from build123d import *

# Parameters (mm, degrees)
F1_DEPTH = 25.4


with BuildPart() as f1:
    # F0 (on Front) → F1 (new body)
    with BuildSketch(Plane.XZ):
        with BuildLine():
            Line((-1.5875, 27.281528), (-2.760676, 25.249528))
            ThreePointArc((-2.760676, 25.249528), (-4.410664, 25.014117), (-6.041661, 24.671002))
            ThreePointArc((-6.041661, 24.671002), (-8.687312, 23.868193), (-11.230034, 22.782589))
            ThreePointArc((-11.230034, 22.782589), (-12.7, 21.997045), (-14.115283, 21.116789))
            ThreePointArc((-14.115283, 21.116789), (-16.326805, 19.457529), (-18.344884, 17.567733))
            ThreePointArc((-18.344884, 17.567733), (-19.457529, 16.326805), (-20.486395, 15.015579))
            ThreePointArc((-20.486395, 15.015579), (-21.997045, 12.7), (-23.247071, 10.233949))
            ThreePointArc((-23.247071, 10.233949), (-23.868193, 8.687312), (-24.386545, 7.103269))
            ThreePointArc((-24.386545, 7.103269), (-25.014117, 4.410664), (-25.345317, 1.6658))
            ThreePointArc((-25.345317, 1.6658), (-25.4, 0), (-25.345317, -1.6658))
            ThreePointArc((-25.345317, -1.6658), (-25.014117, -4.410664), (-24.386545, -7.103269))
            ThreePointArc((-24.386545, -7.103269), (-23.868193, -8.687312), (-23.247071, -10.233949))
            ThreePointArc((-23.247071, -10.233949), (-21.997045, -12.7), (-20.486395, -15.015579))
            ThreePointArc((-20.486395, -15.015579), (-19.457529, -16.326805), (-18.344884, -17.567733))
            ThreePointArc((-18.344884, -17.567733), (-16.326805, -19.457529), (-14.115283, -21.116789))
            ThreePointArc((-14.115283, -21.116789), (-12.7, -21.997045), (-11.230034, -22.782589))
            ThreePointArc((-11.230034, -22.782589), (-8.687312, -23.868193), (-6.041661, -24.671002))
            ThreePointArc((-6.041661, -24.671002), (-4.410664, -25.014117), (-2.760676, -25.249528))
            ThreePointArc((-2.760676, -25.249528), (0, -25.4), (2.760676, -25.249528))
            ThreePointArc((2.760676, -25.249528), (4.410664, -25.014117), (6.041661, -24.671002))
            ThreePointArc((6.041661, -24.671002), (8.687312, -23.868193), (11.230034, -22.782589))
            ThreePointArc((11.230034, -22.782589), (12.7, -21.997045), (14.115283, -21.116789))
            ThreePointArc((14.115283, -21.116789), (16.326805, -19.457529), (18.344884, -17.567733))
            ThreePointArc((18.344884, -17.567733), (19.457529, -16.326805), (20.486395, -15.015579))
            ThreePointArc((20.486395, -15.015579), (21.997045, -12.7), (23.247071, -10.233949))
            ThreePointArc((23.247071, -10.233949), (23.868193, -8.687312), (24.386545, -7.103269))
            ThreePointArc((24.386545, -7.103269), (25.014117, -4.410664), (25.345317, -1.6658))
            ThreePointArc((25.345317, -1.6658), (25.4, 0), (25.345317, 1.6658))
            ThreePointArc((25.345317, 1.6658), (25.014117, 4.410664), (24.386545, 7.103269))
            ThreePointArc((24.386545, 7.103269), (23.868193, 8.687312), (23.247071, 10.233949))
            ThreePointArc((23.247071, 10.233949), (21.997045, 12.7), (20.486395, 15.015579))
            ThreePointArc((20.486395, 15.015579), (19.457529, 16.326805), (18.344884, 17.567733))
            ThreePointArc((18.344884, 17.567733), (16.326805, 19.457529), (14.115283, 21.116789))
            ThreePointArc((14.115283, 21.116789), (12.7, 21.997045), (11.230034, 22.782589))
            ThreePointArc((11.230034, 22.782589), (8.687312, 23.868193), (6.041661, 24.671002))
            ThreePointArc((6.041661, 24.671002), (4.410664, 25.014117), (2.760676, 25.249528))
            Line((2.760676, 25.249528), (1.5875, 27.281528))
            Line((1.5875, 27.281528), (-1.5875, 27.281528))
        make_face()
        with BuildLine():
            ThreePointArc((-11.230034, 22.782589), (-8.687312, 23.868193), (-6.041661, 24.671002))
            Line((-6.041661, 24.671002), (-7.83907, 26.179208))
            Line((-7.83907, 26.179208), (-10.822594, 25.093294))
            Line((-10.822594, 25.093294), (-11.230034, 22.782589))
        make_face()
        with BuildLine():
            ThreePointArc((-18.344884, 17.567733), (-16.326805, 19.457529), (-14.115283, 21.116789))
            Line((-14.115283, 21.116789), (-16.320133, 21.919288))
            Line((-16.320133, 21.919288), (-18.752324, 19.878438))
            Line((-18.752324, 19.878438), (-18.344884, 17.567733))
        make_face()
        with BuildLine():
            Line((7.83907, 26.179208), (6.041661, 24.671002))
            ThreePointArc((6.041661, 24.671002), (8.687312, 23.868193), (11.230034, 22.782589))
            Line((11.230034, 22.782589), (10.822594, 25.093294))
            Line((10.822594, 25.093294), (7.83907, 26.179208))
        make_face()
        with BuildLine():
            ThreePointArc((-23.247071, 10.233949), (-21.997045, 12.7), (-20.486395, 15.015579))
            Line((-20.486395, 15.015579), (-22.832746, 15.015579))
            Line((-22.832746, 15.015579), (-24.420246, 12.265949))
            Line((-24.420246, 12.265949), (-23.247071, 10.233949))
        make_face()
        with BuildLine():
            Line((16.320133, 21.919288), (14.115283, 21.116789))
            ThreePointArc((14.115283, 21.116789), (16.326805, 19.457529), (18.344884, 17.567733))
            Line((18.344884, 17.567733), (18.752324, 19.878438))
            Line((18.752324, 19.878438), (16.320133, 21.919288))
        make_face()
        with BuildLine():
            ThreePointArc((-25.345317, 1.6658), (-25.014117, 4.410664), (-24.386545, 7.103269))
            Line((-24.386545, 7.103269), (-26.591394, 6.30077))
            Line((-26.591394, 6.30077), (-27.142727, 3.174005))
            Line((-27.142727, 3.174005), (-25.345317, 1.6658))
        make_face()
        with BuildLine():
            Line((22.832746, 15.015579), (20.486395, 15.015579))
            ThreePointArc((20.486395, 15.015579), (21.997045, 12.7), (23.247071, 10.233949))
            Line((23.247071, 10.233949), (24.420246, 12.265949))
            Line((24.420246, 12.265949), (22.832746, 15.015579))
        make_face()
        with BuildLine():
            ThreePointArc((-24.386545, -7.103269), (-25.014117, -4.410664), (-25.345317, -1.6658))
            Line((-25.345317, -1.6658), (-27.142727, -3.174005))
            Line((-27.142727, -3.174005), (-26.591394, -6.30077))
            Line((-26.591394, -6.30077), (-24.386545, -7.103269))
        make_face()
        with BuildLine():
            Line((26.591394, 6.30077), (24.386545, 7.103269))
            ThreePointArc((24.386545, 7.103269), (25.014117, 4.410664), (25.345317, 1.6658))
            Line((25.345317, 1.6658), (27.142727, 3.174005))
            Line((27.142727, 3.174005), (26.591394, 6.30077))
        make_face()
        with BuildLine():
            ThreePointArc((-20.486395, -15.015579), (-21.997045, -12.7), (-23.247071, -10.233949))
            Line((-23.247071, -10.233949), (-24.420246, -12.265949))
            Line((-24.420246, -12.265949), (-22.832746, -15.015579))
            Line((-22.832746, -15.015579), (-20.486395, -15.015579))
        make_face()
        with BuildLine():
            Line((27.142727, -3.174005), (25.345317, -1.6658))
            ThreePointArc((25.345317, -1.6658), (25.014117, -4.410664), (24.386545, -7.103269))
            Line((24.386545, -7.103269), (26.591394, -6.30077))
            Line((26.591394, -6.30077), (27.142727, -3.174005))
        make_face()
        with BuildLine():
            ThreePointArc((-14.115283, -21.116789), (-16.326805, -19.457529), (-18.344884, -17.567733))
            Line((-18.344884, -17.567733), (-18.752324, -19.878438))
            Line((-18.752324, -19.878438), (-16.320133, -21.919288))
            Line((-16.320133, -21.919288), (-14.115283, -21.116789))
        make_face()
        with BuildLine():
            Line((24.420246, -12.265949), (23.247071, -10.233949))
            ThreePointArc((23.247071, -10.233949), (21.997045, -12.7), (20.486395, -15.015579))
            Line((20.486395, -15.015579), (22.832746, -15.015579))
            Line((22.832746, -15.015579), (24.420246, -12.265949))
        make_face()
        with BuildLine():
            ThreePointArc((-6.041661, -24.671002), (-8.687312, -23.868193), (-11.230034, -22.782589))
            Line((-11.230034, -22.782589), (-10.822594, -25.093294))
            Line((-10.822594, -25.093294), (-7.83907, -26.179208))
            Line((-7.83907, -26.179208), (-6.041661, -24.671002))
        make_face()
        with BuildLine():
            Line((18.752324, -19.878438), (18.344884, -17.567733))
            ThreePointArc((18.344884, -17.567733), (16.326805, -19.457529), (14.115283, -21.116789))
            Line((14.115283, -21.116789), (16.320133, -21.919288))
            Line((16.320133, -21.919288), (18.752324, -19.878438))
        make_face()
        with BuildLine():
            ThreePointArc((2.760676, -25.249528), (0, -25.4), (-2.760676, -25.249528))
            Line((-2.760676, -25.249528), (-1.5875, -27.281528))
            Line((-1.5875, -27.281528), (1.5875, -27.281528))
            Line((1.5875, -27.281528), (2.760676, -25.249528))
        make_face()
        with BuildLine():
            Line((10.822594, -25.093294), (11.230034, -22.782589))
            ThreePointArc((11.230034, -22.782589), (8.687312, -23.868193), (6.041661, -24.671002))
            Line((6.041661, -24.671002), (7.83907, -26.179208))
            Line((7.83907, -26.179208), (10.822594, -25.093294))
        make_face()
    extrude(amount=F1_DEPTH)


solid = f1.part
The listing builds one solid part. Answer for the finished solid, in the listing's coordinates (mm). A direction names the side the tool comes from. Coordinates: 2 decimals unless noted, no trailing zeros. Write each loop counter-clockwise with the first axis right and the second up, starting at its lowest first coordinate (ties: lowest second). Pieces come first, ordered by that corner, then holes. Notation, with made-up numbers: M 58.25,17.25 L 73.25,17.25 A23 cw 73.25,31.25 Z; hole C -30.75,60 d4. An arc over 180 degrees is marked long. Put each result on its own line as item: value. Start each with the question number.
1. Consider line 1 (Z direction, x = 6, y = -22.5); line 2 (X direction, y = -2.75, z = 0.5); line 3 (Z direction, x = -10, y = -8). Determine where each line is inside the solid, lowest interval first. Write a range as from..to.
2. A cutting plane is placed at A-A on x = -13. Write down the section's boundary in (y, z), then the cut area to 3 significant figures.
3. Which of the six approach directions +Z, -Z, +X, -X, +Y, -Y give full straight-line access (tool end or side, diameter ignored) to faces 1 (the flat face through (-17.52, -12.52, 20.91)), 2 (the cylindrical face through (-4.43, -12.52, -25.01)), 3 (the cylindrical face through (-4.388, -12.522, 25.018))?
4. For a pull along Z with two mould halves and no side action, classify faces 4 (the flat face through (26.23, -12.52, 2.41)), 5 (the cylindrical face through (23.876, -12.522, 8.665)), 6 (the flat face through (-22, -13, 15.016)), 7 (the flat face through (-9.35, -12.52, -25.63)) as pulls with the +Z half, pulls with the -Z half, needs draft (parallel to the pull), parting line crosses it, or undercut.
5. A cutting plane is placed at B-B on z = 9.5. Write down the section's boundary in (x, y).
6. Flat-ended cylindrical pins translate along their axes: P1, Ø3, axis at x = 17.5, y = -16.5, coming from the +Z side; P2, Ø1.2, axis at x = 22, y = -9, coming from the +Z side; P3, Ø1.5, axis at x = 13.5, y = -23, coming from the +Z side; P4, Ø12, axis at x = 21, z = -14, coming from the +Y side. Find the tip coordinate at first contact, or state that the pin passes through.
Resolved:
1. line 1: z = -24.68..24.68
1. line 2: x = -25.4..25.4
1. line 3: z = -25.39..25.39
2. outline: M -25.4,-21.82 L 0,-21.82 L 0,21.82 L -25.4,21.82 Z
2. area: 1,110 mm2
3. face 1: +Z, -X, +Y, -Y
3. face 2: -Z, +Y, -Y
3. face 3: +Z, +Y, -Y
4. face 4: undercut
4. face 5: undercut
4. face 6: pulls with the +Z half
4. face 7: pulls with the -Z half
5. outline: M -23.56,-25.4 L 23.56,-25.4 L 23.56,0 L -23.56,0 Z
6. P1: stops at z = 21.92
6. P2: stops at z = 15.02
6. P3: stops at z = 21.97
6. P4: stops at y = 0
